Source: CAD feature listing. Evaluate the final solid. Frame: model axes, mm. Face numbers are marked on the shaded views. Round coordinates to 2 decimals unless told otherwise and drop trailing zeros. Loops run counter-clockwise (first coordinate to the right, second up) from the corner with the lowest first, then second, coordinate; pieces in that order, holes last. Notation, with made-up numbers: M 68.25,41 L 120.25,41 A21 ccw 120.25,54 Z; hole C -15,58.25 d1. An arc over 180 degrees is marked long. Answer as CSV lines item,"result". Start each with the question number.
```python
from build123d import *

# Parameters (mm, degrees)
CUT_EXTRUDE1_DEPTH   = 5
SKETCH6_R            = 10.5
CUT_EXTRUDE2_DEPTH   = 5
CUT_EXTRUDE3_DEPTH   = 45
SKETCH8_R            = 40
CUT_EXTRUDE4_DEPTH   = 32
SKETCH9_R            = 34
SKETCH9_R_2          = 24.5
CUT_EXTRUDE5_DEPTH   = 18
SKETCH10_R           = 27
CUT_EXTRUDE6_DEPTH   = 14
INTERSECT1_START     = 14
INTERSECT1_OUTLINE_R = 42
INTERSECT1_DEPTH     = 48


# Read off the part's stored shape, not the designer's step: Intersect1
with BuildPart() as part:
    # Sketch1 → Revolve1 (revolve)
    with BuildSketch(Plane.XY, mode=Mode.PRIVATE) as revolve1_sk:
        with BuildLine():
            Line((22.5, 0), (34, 0))
            ThreePointArc((34, 0), (35.414213562, 0.585786438), (36, 2))
            Line((36, 2), (36, 20))
            Line((36, 20), (40, 20))
            ThreePointArc((40, 20), (41.414213562, 20.585786438), (42, 22))
            Line((42, 22), (42, 57))
            ThreePointArc((42, 57), (40.535533906, 60.535533906), (37, 62))
            Line((37, 62), (0, 62))
            Line((0, 62), (0, 20))
            Line((0, 20), (22.5, 20))
            Line((22.5, 20), (22.5, 0))
        make_face()
    revolve(revolve1_sk.sketch.rotate(Axis((0, 2, 0), (0, 1, 0)), 90), axis=Axis((0, 2, 0), (0, 1, 0)))

    # Sketch5 → Cut-Extrude1 (cut)
    with BuildSketch(Plane(origin=(0, 62, 0), x_dir=(1, 0, 0), z_dir=(0, 1, 0))):
        with BuildLine():
            Line((-42, 0), (-40, 0))
            Line((-40, 0), (40, 0))
            Line((40, 0), (42, 0))
            ThreePointArc((42, 0), (0, 42), (-42, 0))
        make_face()
    extrude(amount=-CUT_EXTRUDE1_DEPTH, mode=Mode.SUBTRACT)

    # Sketch6 → Cut-Extrude2 (cut)
    with BuildSketch(Plane.XY.offset(42)):
        with Locations((-2, 42)):
            Circle(SKETCH6_R)
    extrude(amount=-CUT_EXTRUDE2_DEPTH, mode=Mode.SUBTRACT)

    # Sketch7 → Cut-Extrude3 (cut)
    with BuildSketch(Plane.XZ.offset(-20)):
        with BuildLine():
            Line((-21, 0), (21, 0))
            ThreePointArc((21, 0), (0, -21), (-21, 0))
        make_face()
    extrude(amount=-CUT_EXTRUDE3_DEPTH, mode=Mode.SUBTRACT)

    # Sketch8 → Cut-Extrude4 (cut)
    with BuildSketch(Plane(origin=(0, 54.5, 0), x_dir=(1, 0, 0), z_dir=(0, 1, 0))):
        with Locations(Location((0, 0, 0), (0, 0, 270))):
            Circle(SKETCH8_R)
        with BuildLine():
            Line((22.912878475, -2), (-22.912878475, -2))
            ThreePointArc((-22.912878475, -2), (0, 23), (22.912878475, -2))
        make_face(mode=Mode.SUBTRACT)
    extrude(amount=-CUT_EXTRUDE4_DEPTH, mode=Mode.SUBTRACT)

    # Sketch9 → Cut-Extrude5 (cut)
    with BuildSketch(Plane(origin=(0, 2, 0), x_dir=(-1, 0, 0), z_dir=(0, -1, 0))):
        with Locations(Location((0, 0, 0), (0, 0, 90))):
            Circle(SKETCH9_R)
        with Locations(Location((0, 0, 0), (0, 0, 90))):
            Circle(SKETCH9_R_2, mode=Mode.SUBTRACT)
    extrude(amount=-CUT_EXTRUDE5_DEPTH, mode=Mode.SUBTRACT)

    # Sketch10 → Cut-Extrude6 (cut)
    with BuildSketch(Plane(origin=(0, 2, 0), x_dir=(-1, 0, 0), z_dir=(0, -1, 0))):
        Circle(SKETCH10_R)
    extrude(amount=-CUT_EXTRUDE6_DEPTH, mode=Mode.SUBTRACT)

    # Intersect1 outline → Intersect1 (cut)
    with BuildSketch(Plane(origin=(0, 0, 0), x_dir=(1, 0, 0), z_dir=(0, 1, 0)).offset(INTERSECT1_START)):
        Circle(INTERSECT1_OUTLINE_R)
        with BuildLine():
            ThreePointArc((-21, 0), (0, 21), (21, 0))
            Line((21, 0), (-21, 0))
        make_face(mode=Mode.SUBTRACT)
    extrude(amount=INTERSECT1_DEPTH, mode=Mode.SUBTRACT)


solid = part.part
```
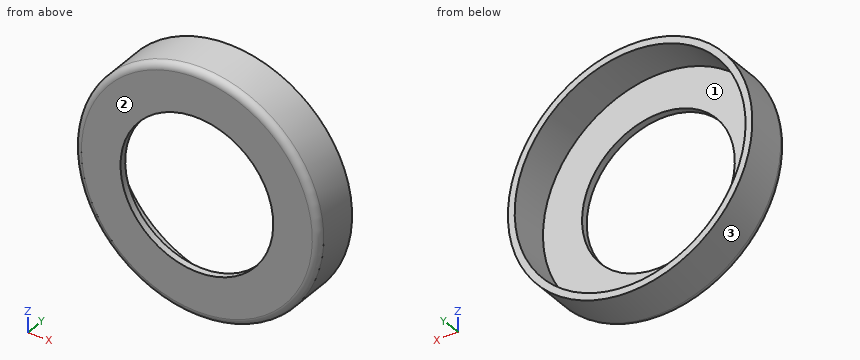
1) Section B-B, the plane z = 0. Return loops of the section in (x, y), and give its area (3 significant figures).
2) Mould query, pull axis Z, two halves, no side actions, for the marked faces 1, 2 and 3. Classes: pulls with the +Z half, pulls with the -Z half, needs draft (parallel to the pull), parting line crosses it, or undercut.
3) Section C-C, the plane y = 10. Return loops of the section in (x, z).
4) Ray query, line 1 along X through (y, z) = (9.25, 0); line 2 along Y through (x, z) = (20.5, -27); line 3 along X through (y, z) = (7.25, -20). Return the intervals inside material, ascending.
5) Section D-D, the plane y = 1. Return loops of the section in (x, z).
6) Section A-A, the plane x = 0. Return loops of the section in (y, z).
7) Contact query for flat-ended pins moving along their axis: pin 1 Ø3 at (y, z) = (11.5, 6.5) entering from -X; pin 2 Ø6 at (x, y) = (10.5, 5) entering from -Z; pin 3 Ø8 at (y, z) = (2.5, -9.5) entering from +X. Output: stop coordinate, or through.
Findings below:
1,outline,"M -36,2 A2 ccw -34,0 L -22.5,0 L -22.5,2 L -34,2 L -34,14 L -36,14 Z; M 22.5,0 L 34,0 A2 ccw 36,2 L 36,14 L 34,14 L 34,2 L 22.5,2 Z"
1,area,"100 mm²"
2,face 1,"undercut"
2,face 2,"needs draft"
2,face 3,"parting line crosses it"
3,outline,"C 0,0 d72; hole C 0,0 d68"
4,line 1,"-36 to -34, 34 to 36"
4,line 2,"0 to 2"
4,line 3,"-29.93 to -27.5, 27.5 to 29.93"
5,outline,"C 0,0 d71.46; hole C 0,0 d45"
6,outline,"M 0,-34 A2 ccw 2,-36 L 14,-36 L 14,-34 L 2,-34 L 2,-22.5 L 0,-22.5 Z; M 0,22.5 L 2,22.5 L 2,34 L 14,34 L 14,36 L 2,36 A2 ccw 0,34 Z"
7,pin 1,"x = -35.65"
7,pin 2,"z = -35.21"
7,pin 3,"x = 35.58"
